Here's how the part is built. I have some questions about the finished solid (model axes, mm). A direction names the side the tool comes from. Coordinates: 2 decimals unless noted, no trailing zeros. Write each loop counter-clockwise with the first axis right and the second up, starting at its lowest first coordinate (ties: lowest second). Pieces come first, ordered by that corner, then holes.
(1) For pin 1 Ø3.5 at (x, y) = (-25, 7.5) entering from +Z; pin 2 Ø2 at (x, y) = (-28.5, 12) entering from +Z, each with a flat end and sliding along its axis, tell me the tip position at first contact or that it passes through.
(2) Imagine slicing it at D-D, the plane z = 5.6. List the corners of the cut face in (x, y) for me, plus the area to 3 significant figures.
(3) Please list where these lines run through material, in increasing order: probe 1 along X at (y, z) = (9.25, 3.05); probe 2 along Y at (x, z) = (-22.75, 4.3); probe 3 along X at (y, z) = (8.5, 5.05).
(4) Imagine slicing it at C-C, the plane y = 1.75. List the corners of the cut face in (x, z) for me.
(5) Imagine slicing it at A-A, the plane x = -29.5. List the corners of the cut face in (y, z) for me.
(6) Thinking about a two-plate mould opening in X: for faces 1 (the cylindrical face through (-25.32, 9.46, 3.24)), 2 (the flat face through (-34, 13, 4.98)), 3 (the cylindrical face through (-34.44, 5.69, 3.72)), which applies, released by +X, released by -X, zero draft, split by the parting line, or undercut?
(7) Imagine slicing it at B-B, the plane z = 2.8. List the corners of the cut face in (x, y) for me.
(8) Which directions (+Z, -Z, +X, -X, +Y, -Y) give clear straight access to the entire face, cutting with the end or side of a thin tool? Please do faces 4 (the flat face through (-20, 9, 2.5)), 5 (the flat face through (-20, 9, 4)).
```python
from build123d import *

# Parameters (mm, degrees)
EXTRUDE_START       = 2.5
SKETCH_1_R          = 12.2
EXTRUDE_1_DEPTH     = 2.48
EXTRUDE_START_2     = 4.98
SKETCH_2_R          = 11.35
EXTRUDE_2_DEPTH     = 2.02
CUT_EXTRUDE_START   = 7
SKETCH_3_R          = 6.15
CUT_EXTRUDE_1_DEPTH = 3
CHAMFER_1_SIZE      = 0.2
CUT_EXTRUDE_START_2 = 2.5
SKETCH_4_R          = 2.52
CUT_EXTRUDE_2_DEPTH = 1.5


with BuildPart() as part:
    # 草图1 → 凸台-拉伸1 (new body)
    with BuildSketch(Plane.XY.offset(EXTRUDE_START)):
        with Locations(Location((-22.803986485, 9.350307143, 0), (0, 0, 180))):
            Circle(SKETCH_1_R)
    extrude(amount=EXTRUDE_1_DEPTH)

    # 草图2 → 凸台-拉伸2 (add)
    with BuildSketch(Plane.XY.offset(EXTRUDE_START_2)):
        with Locations(Location((-22.803986485, 9.350307143, 0), (0, 0, 270))):
            Circle(SKETCH_2_R)
    extrude(amount=EXTRUDE_2_DEPTH)

    # 草图3 → 切除-拉伸1 (cut)
    with BuildSketch(Plane.XY.offset(CUT_EXTRUDE_START)):
        with Locations((-22.803986485, 9.350307143)):
            Circle(SKETCH_3_R)
    extrude(amount=-CUT_EXTRUDE_1_DEPTH, mode=Mode.SUBTRACT)

    # 倒角1
    chamfer_1_edges = [part.edges().sort_by_distance(p)[0] for p in [
        (-28.953986485, 9.350307143, 7),
    ]]
    chamfer(chamfer_1_edges, length=CHAMFER_1_SIZE)

    # 草图4 → 切除-拉伸2 (cut)
    with BuildSketch(Plane.XY.offset(CUT_EXTRUDE_START_2)):
        with Locations((-22.803986485, 9.350307143)):
            Circle(SKETCH_4_R)
    extrude(amount=CUT_EXTRUDE_2_DEPTH, mode=Mode.SUBTRACT)


solid = part.part
```
Recorded:
1. pin 1: stops at z = 4
1. pin 2: stops at z = 7
2. outline: circle Ø22.7 at (-22.8, 9.35); hole circle Ø12.3 at (-22.8, 9.35)
2. area: 286 mm2
3. probe 1: x = -35 to -25.32, -20.29 to -10.6
3. probe 2: y = -2.85 to 3.2, 15.5 to 21.55
3. probe 3: x = -34.12 to -28.89, -16.71 to -11.49
4. outline: (-32.35, 2.5) - (-13.26, 2.5) - (-13.26, 4.98) - (-14.37, 4.98) - (-14.37, 7) - (-31.23, 7) - (-31.23, 4.98) - (-32.35, 4.98) - close
5. outline: (-0.85, 2.5) - (19.55, 2.5) - (19.55, 4.98) - (18.51, 4.98) - (18.51, 7) - (0.19, 7) - (0.19, 4.98) - (-0.85, 4.98) - close
6. face 1: undercut
6. face 2: zero draft
6. face 3: split by the parting line
7. outline: circle Ø24.4 at (-22.8, 9.35); hole circle Ø5.04 at (-22.8, 9.35)
8. face 4: -Z, +X, -X, +Y, -Y
8. face 5: +Z
